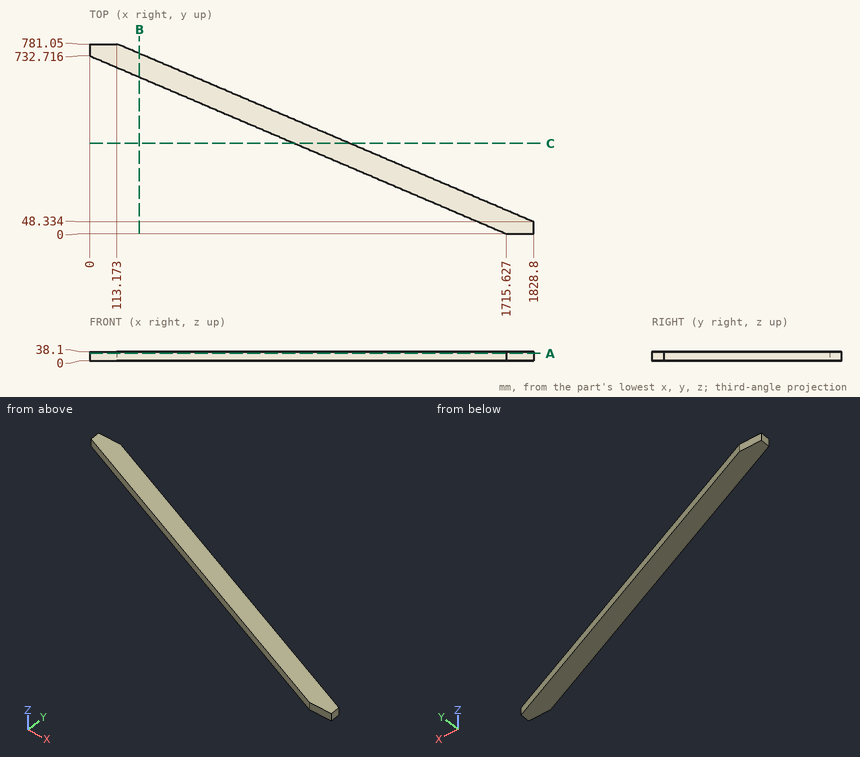
Check sheet for the drawn part. Datum: minimum x, y, z corner. Units: mm. Round coordinates to 2 decimals unless told otherwise and drop trailing zeros. Loops run counter-clockwise (first coordinate to the right, second up) from the corner with the lowest first, then second, coordinate; pieces in that order, holes last. Notation, with made-up numbers: M 56,58 L 106,58 A33 ccw 106,94 Z; hole C 34,30.25 d8. An arc over 180 degrees is marked long. One line per question, with ' | ' between items. Start each with the question number.
Item 1: Section check B-B (x = 205). Record the boundary of the cut face in (y, z), and give its area (3 significant figures).
Item 2: Section check A-A (z = 31). Record the boundary of the cut face in (x, y), and give its area (3 significant figures).
Item 3: Scan lines: probe 1 along Y at (x, z) = (1223.5, 15); probe 2 along X at (y, z) = (136, 26) (1 decimal); probe 3 along Y at (x, z) = (1188, 24). Record each from-to range of solid material in increasing order.
Item 4: Section check C-C (y = 372). Record the boundary of the cut face in (x, z), and give its area (3 significant figures).
Item 5: Gauge pin test, flat ends, axial feed: pin 1 Ø1.5 at (y, z) = (573, 22.5) entering from +X; pin 2 Ø4 at (y, z) = (309.5, 18) entering from -X; pin 3 Ø5 at (x, z) = (454.5, 12) entering from -Y. Record the tip position at first contact, or that the pin passes through.
Worked out:
1) outline: M 645.16,0 L 741.83,0 L 741.83,38.1 L 645.16,38.1 Z | area: 3,680 mm^2
2) outline: M 0,732.72 L 1715.63,0 L 1828.8,0 L 1828.8,48.33 L 113.17,781.05 L 0,781.05 Z | area: 171,000 mm^2
3) probe 1: 210.18 to 306.85 | probe 2: 1397.2 to 1623.5 | probe 3: 225.34 to 322.01
4) outline: M 844.6,0 L 1070.95,0 L 1070.95,38.1 L 844.6,38.1 Z | area: 8,620 mm^2
5) pin 1: x = 602.07 | pin 2: x = 986.26 | pin 3: y = 537.54
